Could you check a few things on this model? Use its own coordinates, in mm. Face numbers are marked on the shaded views. A direction names the side the tool comes from. Round coordinates to 2 decimals unless told otherwise and drop trailing zeros. Loops run counter-clockwise (first coordinate to the right, second up) from the corner with the lowest first, then second, coordinate; pieces in that order, holes last. Notation, with made-up numbers: (27, 19.25) -> (43, 19.25) arc R17 cw to (43, 45.25) -> close; hole circle Ø11 at (46, 42). An arc over 180 degrees is marked (long way). One line per item, written item: value.
```python
from build123d import *

# Parameters (mm, degrees)
F0_R     = 3.175
F1_DEPTH = 31.75
F2_R     = 12.7
F3_DEPTH = 144.018


with BuildPart() as f1:
    # F0 (on Front) → F1 (new body)
    with BuildSketch(Plane.XZ):
        with BuildLine():
            ThreePointArc((-48.26, -15.862295), (8.032185, -50.160981), (50.8, 0))
            ThreePointArc((50.8, 0), (8.032185, 50.160981), (-48.26, 15.862295))
            Line((-48.26, 15.862295), (-48.26, -15.862295))
        make_face()
        Circle(F0_R, mode=Mode.SUBTRACT)
    extrude(amount=F1_DEPTH)

    # F2 (on face) → F3 (join)
    with BuildSketch(Plane(origin=(-48.26, 0, 0), x_dir=(0, -1, 0), z_dir=(-1, 0, 0))):
        with Locations((15.875, 0)):
            Circle(F2_R)
    extrude(amount=F3_DEPTH)


solid = f1.part
```
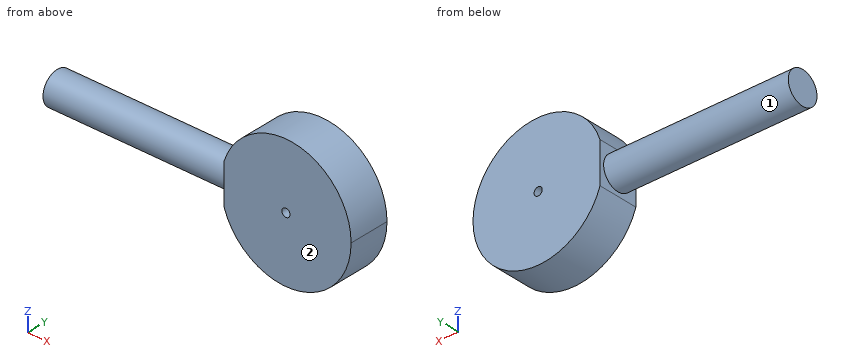
(1) Imagine slicing it at D-D on x = -136. Write out the boundary of the cut face in (y, z) (3 decimals), then the cut area to 3 significant figures.
Results below:
outline: circle Ø25.4 at (-15.875, 0)
area: 507 mm²
(2) Imagine slicing it at A-A on x = 0. Write out the boundary of the cut face in (y, z) (3 decimals).
Results below:
outline: (-31.75, -50.8) -> (0, -50.8) -> (0, -3.175) -> (-31.75, -3.175) -> close; (-31.75, 3.175) -> (0, 3.175) -> (0, 50.8) -> (-31.75, 50.8) -> close
(3) Please list where these lines run through material, in increasing order: L1, parallel to X at y = -10, z = -0.5; L2, parallel to Z at x = 0, y = -15.5 (3 decimals); L3, parallel to X at y = -10, z = 1.5.
Results below:
L1: x = -192.28 to -3.14, 3.14 to 50.8
L2: z = -50.8 to -3.175, 3.175 to 50.8
L3: x = -192.28 to -2.8, 2.8 to 50.78
(4) On a 3-axis mill with a long thin cutter (end or side, diameter ignored), from which of +Z, -Z, +X, -X, +Y, -Y can I reach the whole of each face in a straight line? I mean the marked faces 1 and 2. Say none if no direction works.
Results below:
face 1: -X
face 2: +Z, -Z, +X, -X, -Y
(5) Imagine slicing it at C-C on z = 6. Write out the boundary of the cut face in (x, y).
Results below:
outline: (-192.28, -27.07) -> (-48.26, -27.07) -> (-48.26, -31.75) -> (50.44, -31.75) -> (50.44, 0) -> (-48.26, 0) -> (-48.26, -4.68) -> (-192.28, -4.68) -> close
(6) For pin 1 Ø5 at (y, z) = (-17.5, 23) entering from -X; pin 2 Ø10 at (x, y) = (-166.5, -15) entering from +Z; pin 3 Ø2 at (y, z) = (-9, 21) entering from -X, each with a flat end and sliding along its axis, tell me the tip position at first contact or that it passes through.
Results below:
pin 1: stops at x = -46.48
pin 2: stops at z = 12.7
pin 3: stops at x = -46.7
(7) Imagine slicing it at B-B on y = -12.5. Write out the boundary of the cut face in (x, z) (3 decimals).
Results below:
outline: (-192.278, -12.243) -> (-48.26, -12.243) -> (-48.26, -15.862) arc R50.8 ccw (long way) to (-48.26, 15.862) -> (-48.26, 12.243) -> (-192.278, 12.243) -> close; hole circle Ø6.35 at (0, 0)
